Check sheet for the modelled part. Datum: model origin and axes. Units: mm. A direction names the side the tool comes from. Round coordinates to 2 decimals unless told otherwise and drop trailing zeros. Loops run counter-clockwise (first coordinate to the right, second up) from the corner with the lowest first, then second, coordinate; pieces in that order, holes last. Notation, with made-up numbers: (78, 77) -> (132, 77) arc R27 ccw to (132, 93) -> close; hole circle Ø10 at (3, 8). An arc over 180 degrees is marked (long way). Use one line per item in the form item = value. Start each with the question number.
(1) Sectioned sample at A-A (y = 0). Record the cut outline in (x, z), and give its area (3 significant figures).
(2) Set-up check for faces 5 (the cylindrical face through (-1.65, -7.44, 6.98)), 6 (the flat face through (-11, 6.35, 4)), 7 (the flat face through (0, 8, 6.35)): record each of +Z, -Z, +X, -X, +Y, -Y from which the full face is reachable in a straight line by a thin tool's end or side.
(3) Draft check along Z on faces 1 (the flat face through (12.741, 0, 4)), 2 (the flat face through (0, 0, 0)), 3 (the flat face through (0, 8, 7.62)), 4 (the flat face through (0, 0, 0.762)). Enter one of: released by +Z, released by -Z, zero draft, split by the parting line, or undercut.
(4) Sectioned sample at D-D (x = 8.5). Record the cut outline in (y, z), and give its area (3 significant figures).
(5) Sectioned sample at C-C (x = 0). Record the cut outline in (y, z).
(6) Go/stop test with a flat-tipped pin: pin 1 (5.5 mm diameter, centred on x = 1, y = 4, fed in from +Z). Record where the tip stops, or that it passes through.
(7) Material ranges on probe 1 along Z at (x, y) = (-1.25, 9.25); probe 2 along X at (y, z) = (-3.75, 6.5); probe 3 along Y at (x, z) = (-5.5, 4), recorded low to high. Write a range as [from, to].
(8) Sectioned sample at B-B (z = 4.75). Record the cut outline in (x, y), and give its area (3 significant figures).
from build123d import *

# Parameters (mm, degrees)
SKETCH1_W           = 27.94
SKETCH1_H           = 22.86
BOSS_EXTRUDE1_DEPTH = 6.35
SKETCH2_R           = 9.398
CUT_EXTRUDE1_DEPTH  = 5.588
SKETCH3_W           = 27.94
SKETCH3_H           = 22.86
SKETCH3_R           = 7.62
BOSS_EXTRUDE2_DEPTH = 1.27
SKETCH9_W           = 2.54
SKETCH9_H           = 12.7
CUT_EXTRUDE3_DEPTH  = 7.62


with BuildPart() as part:
    # Sketch1 → Boss-Extrude1 (new body)
    with BuildSketch(Plane.XY):
        Rectangle(SKETCH1_W, SKETCH1_H)
    extrude(amount=BOSS_EXTRUDE1_DEPTH)

    # Sketch2 → Cut-Extrude1 (cut)
    with BuildSketch(Plane.XY.offset(6.35)):
        Circle(SKETCH2_R)
    extrude(amount=-CUT_EXTRUDE1_DEPTH, mode=Mode.SUBTRACT)

    # Sketch3 → Boss-Extrude2 (add)
    with BuildSketch(Plane.XY.offset(6.35)):
        Rectangle(SKETCH3_W, SKETCH3_H)
        Circle(SKETCH3_R, mode=Mode.SUBTRACT)
    extrude(amount=BOSS_EXTRUDE2_DEPTH)

    # Sketch9 → Cut-Extrude3 (cut)
    with BuildSketch(Plane.XY.offset(7.62)):
        with Locations((-11.47066929, 0)):
            Rectangle(SKETCH9_W, SKETCH9_H)
        with Locations((11.47066929, 0)):
            Rectangle(SKETCH9_W, SKETCH9_H)
    extrude(amount=-CUT_EXTRUDE3_DEPTH, mode=Mode.SUBTRACT)


solid = part.part
Checks:
q1.outline = (-13.97, 0) -> (-12.74, 0) -> (-12.74, 7.62) -> (-13.97, 7.62) -> close; (-10.2, 0) -> (10.2, 0) -> (10.2, 7.62) -> (7.62, 7.62) -> (7.62, 6.35) -> (9.4, 6.35) -> (9.4, 0.76) -> (-9.4, 0.76) -> (-9.4, 6.35) -> (-7.62, 6.35) -> (-7.62, 7.62) -> (-10.2, 7.62) -> close; (12.74, 0) -> (13.97, 0) -> (13.97, 7.62) -> (12.74, 7.62) -> close
q1.area = 49.8 mm2
q2.face_5 = +Z
q2.face_6 = +Z, -Z
q2.face_7 = none
q3.face_1 = zero draft
q3.face_2 = released by -Z
q3.face_3 = released by +Z
q3.face_4 = undercut
q4.outline = (-11.43, 0) -> (11.43, 0) -> (11.43, 7.62) -> (-11.43, 7.62) -> close; hole (-4.01, 0.76) -> (4.01, 0.76) -> (4.01, 6.35) -> (-4.01, 6.35) -> close
q4.area = 129 mm2
q5.outline = (-11.43, 0) -> (11.43, 0) -> (11.43, 7.62) -> (7.62, 7.62) -> (7.62, 6.35) -> (9.4, 6.35) -> (9.4, 0.76) -> (-9.4, 0.76) -> (-9.4, 6.35) -> (-7.62, 6.35) -> (-7.62, 7.62) -> (-11.43, 7.62) -> close
q6.pin_1 = 0.76
q7.probe_1 = [0, 0.76], [6.35, 7.62]
q7.probe_2 = [-13.97, -12.74], [-10.2, -6.63], [6.63, 10.2], [12.74, 13.97]
q7.probe_3 = [-11.43, -7.62], [7.62, 11.43]
q8.outline = (-13.97, -11.43) -> (13.97, -11.43) -> (13.97, 11.43) -> (-13.97, 11.43) -> close; hole (-12.74, -6.35) -> (-10.2, -6.35) -> (-10.2, 6.35) -> (-12.74, 6.35) -> close; hole circle Ø18.8 at (0, 0); hole (10.2, -6.35) -> (12.74, -6.35) -> (12.74, 6.35) -> (10.2, 6.35) -> close
q8.area = 297 mm2
